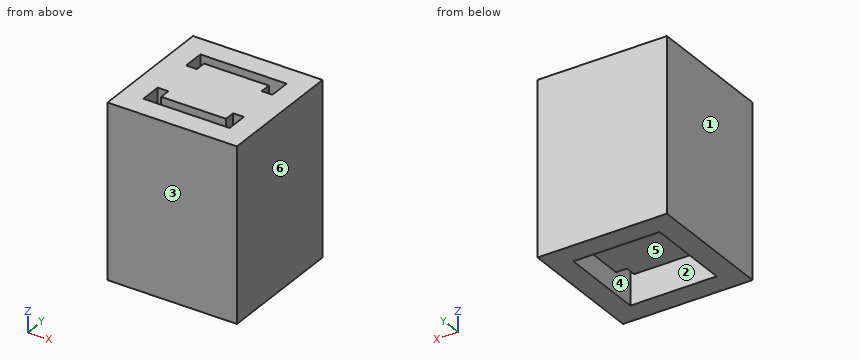
```python
from build123d import *

# Parameters (mm, degrees)
F0_W     = 30
F0_H     = 30
F0_W_2   = 15
F0_H_2   = 10
F0_H_3   = 2.5
F0_W_3   = 2.5
F1_DEPTH = 40
F2_DEPTH = 5
F3_DEPTH = 40


with BuildPart() as f1:
    # F0 (on Top) → F1 (new body)
    with BuildSketch(Plane.XY):
        Rectangle(F0_W, F0_H)
        Polygon((10, 5), (10, -5), (10, -10), (-10, -10), (-10, -5), (-10, 5), (-10, 10), (10, 10), align=None, mode=Mode.SUBTRACT)
        Rectangle(F0_W_2, F0_H_2)
        Polygon((7.5, 7.5), (7.5, 5), (10, 5), (10, 10), (-10, 10), (-10, 5), (-7.5, 5), (-7.5, 7.5), align=None)
        Polygon((7.5, -5), (7.5, -7.5), (-7.5, -7.5), (-7.5, -5), (-10, -5), (-10, -10), (10, -10), (10, -5), align=None)
        with Locations((0, 6.25)):
            Rectangle(F0_W_2, F0_H_3)
        with Locations((0, -6.25)):
            Rectangle(F0_W_2, F0_H_3)
        with Locations((8.75, 0)):
            Rectangle(F0_W_3, F0_H_2)
        with Locations((-8.75, 0)):
            Rectangle(F0_W_3, F0_H_2)
    extrude(amount=F1_DEPTH)

    # F0 (on Top) → F2 (cut)
    with BuildSketch(Plane.XY):
        with Locations((0, -6.25)):
            Rectangle(F0_W_2, F0_H_3)
        Rectangle(F0_W_2, F0_H_2)
        with Locations((0, 6.25)):
            Rectangle(F0_W_2, F0_H_3)
        with Locations((8.75, 0)):
            Rectangle(F0_W_3, F0_H_2)
        with Locations((-8.75, 0)):
            Rectangle(F0_W_3, F0_H_2)
    extrude(amount=F2_DEPTH, mode=Mode.SUBTRACT)

    # F0 (on Top) → F3 (cut)
    with BuildSketch(Plane.XY):
        Polygon((7.5, -5), (7.5, -7.5), (-7.5, -7.5), (-7.5, -5), (-10, -5), (-10, -10), (10, -10), (10, -5), align=None)
        Polygon((7.5, 7.5), (7.5, 5), (10, 5), (10, 10), (-10, 10), (-10, 5), (-7.5, 5), (-7.5, 7.5), align=None)
    extrude(amount=F3_DEPTH, mode=Mode.SUBTRACT)


solid = f1.part
```
Verification items for the finished model (mm, model axes). Face numbers are marked on the shaded views. A direction names the side the tool comes from. Round coordinates to 2 decimals unless told otherwise and drop trailing zeros. Write each loop counter-clockwise with the first axis right and the second up, starting at its lowest first coordinate (ties: lowest second). Pieces come first, ordered by that corner, then holes.
1. Access from +Z, -Z, +X, -X, +Y, -Y to the whole of each face (thin tool, end or side, straight path). Record for the marked faces 5 and 6.
2. Gauge pin test, flat ends, axial feed: P1, Ø3, axis at x = 3, y = 11.5, coming from the -Z side; P2, Ø16.5, axis at x = 1, y = 0.5, coming from the -Z side. Record the tip position at first contact, or that the pin passes through.
3. Section check B-B on y = -8.5. Enter the section's corners in (x, z).
4. Scan lines: L1, parallel to Y at x = 3.5, z = 37; L2, parallel to Y at x = -9, z = 20.5. Record each from-to range of solid material in increasing order.
5. Section check C-C on z = 22. Enter the section's corners in (x, y), plus the area to 3 significant figures.
6. Section check A-A on x = 8.25. Enter the section's corners in (y, z), plus the area to 3 significant figures.
7. Section check D-D on y = 6.75. Enter the section's corners in (x, z), plus the area to 3 significant figures.
8. Draft check along X on the marked faces 1, 2, 3 and 4. Enter one of: +X half, -X half, draft (parallel to the pull), parting line (faces both ways), or undercut.
Answer:
1. face 5: -Z
1. face 6: +Z, -Z, +X, +Y, -Y
2. P1: stops at z = 0
2. P2: stops at z = 5
3. outline: (-15, 0) - (-10, 0) - (-10, 40) - (-15, 40) - close; (10, 0) - (15, 0) - (15, 40) - (10, 40) - close
4. L1: y = -15 to -10, -7.5 to 7.5, 10 to 15
4. L2: y = -15 to -10, -5 to 5, 10 to 15
5. outline: (-15, -15) - (15, -15) - (15, 15) - (-15, 15) - close; hole (-10, -10) - (10, -10) - (10, -5) - (7.5, -5) - (7.5, -7.5) - (-7.5, -7.5) - (-7.5, -5) - (-10, -5) - close; hole (-10, 5) - (-7.5, 5) - (-7.5, 7.5) - (7.5, 7.5) - (7.5, 5) - (10, 5) - (10, 10) - (-10, 10) - close
5. area: 775 mm2
6. outline: (-15, 0) - (-10, 0) - (-10, 40) - (-15, 40) - close; (-5, 5) - (5, 5) - (5, 40) - (-5, 40) - close; (10, 0) - (15, 0) - (15, 40) - (10, 40) - close
6. area: 750 mm2
7. outline: (-15, 0) - (-10, 0) - (-10, 40) - (-15, 40) - close; (-7.5, 5) - (7.5, 5) - (7.5, 40) - (-7.5, 40) - close; (10, 0) - (15, 0) - (15, 40) - (10, 40) - close
7. area: 925 mm2
8. face 1: -X half
8. face 2: undercut
8. face 3: draft
8. face 4: undercut
